```python
from build123d import *

# Parameters (mm, degrees)
SKETCH056_W             = 126
SKETCH056_H             = 25
SKETCH056_R             = 2.2
PAD024_DEPTH            = 3
SKETCH057_W             = 12.4
SKETCH057_H             = 4
PAD025_DEPTH            = 21.5
SKETCH058_R             = 2.2
POCKET031_DEPTH         = 10.609
CHAMFER023_SIZE         = 1
BODY012_ROLL_ANGLE      = 90
BODY012_PLACEMENT_ANGLE = 180


with BuildPart() as part:
    # Sketch056 → Pad024 (new body)
    with BuildSketch(Plane.XY):
        Rectangle(SKETCH056_W, SKETCH056_H)
        with Locations((-53, 0.726)):
            Circle(SKETCH056_R, mode=Mode.SUBTRACT)
        with Locations((53, 0.726)):
            Circle(SKETCH056_R, mode=Mode.SUBTRACT)
    extrude(amount=PAD024_DEPTH)

    # Sketch057 (on Face8 of Pad024) → Pad025 (join)
    with BuildSketch(Plane.XY.offset(3)):
        with Locations((-38.154, -3.892)):
            Rectangle(SKETCH057_W, SKETCH057_H)
        with Locations((38.154, -3.892)):
            Rectangle(SKETCH057_W, SKETCH057_H)
    extrude(amount=PAD025_DEPTH)

    # Sketch058 (on Face12 of Pad025) → Pocket031 (cut, through all)
    with BuildSketch(Plane(origin=(0, -1.892, 0), x_dir=(-1, 0, 0), z_dir=(0, 1, 0))):
        with Locations((-38.154, 18.3)):
            Circle(SKETCH058_R)
        with Locations((38.154, 18.3)):
            Circle(SKETCH058_R)
    extrude(amount=-POCKET031_DEPTH, mode=Mode.SUBTRACT)

    # Chamfer023
    chamfer023_edges = [part.edges().sort_by_distance(p)[0] for p in [
        (0, 12.5, 0),
        (63, 0, 0),
        (0, -12.5, 0),
        (-63, 0, 0),
        (50.8, 0.726, 0),
        (-55.2, 0.726, 0),
    ]]
    chamfer(chamfer023_edges, length=CHAMFER023_SIZE)


with BuildPart() as part_1:
    # Body012 roll: moved
    add(part.part.rotate(Axis((0, 0, 0), (1, 0, 0)), BODY012_ROLL_ANGLE))


with BuildPart() as part_2:
    # Body012 placement: moved
    add(part_1.part.moved(Location((0, -143.1, -77.85))).rotate(Axis((0, -143.1, -77.85), (0, 0, 1)), BODY012_PLACEMENT_ANGLE))


solid = part_2.part
```
Input: part model. Units: mm. Frame: model coordinates. A direction names the side the tool comes from. Round coordinates to 2 decimals unless told otherwise and drop trailing zeros. Order: outer loops, then holes, each group sorted by start corner. A loop starts at its lowest first (then second) coordinate and runs counter-clockwise, first axis right, second up. Notation, with made-up numbers: (58.5, -35.75) - (87.5, -35.75) arc R25 cw to (87.5, -0.75) - close; hole circle Ø7 at (67, 51). An arc over 180 degrees is marked (long way). One line per question, with ' | ' between items. Start each with the question number.
1) Contact query for flat-ended pins moving along their axis: P1, Ø4.5, axis at y = -130.5, z = -81, coming from the -X side; P2, Ø5.5, axis at x = -38.154, y = -124.8, coming from the +Z side; P3, Ø5.5, axis at x = 53, z = -77.124, coming from the +Y side; P4, Ø2, axis at y = -122, z = -86.5, coming from the -X side. Output: stop coordinate, or through.
2) Pull-direction query (Y, two-part tool) for faces 1 (the cylindrical face through (36.41, -126.14, -81.71)), 2 (the cylindrical face through (-40.35, -124.7, -81.71)), 3 (the flat face through (-38, -118.6, -82)), 4 (the cylindrical face through (53.48, -141.11, -79.27)); classes: +Y half, -Y half, draft (parallel to the pull), parting line (faces both ways), or undercut.
3) Cut plane C-C, the plane z = -81.75. Return the cut outline in (x, y), then the cut area to 3 significant figures.
4) Set-up query: faces 5 (the flat face through (38, -130, -83.742)), 6 (the flat face through (38, -130, -79.742)), 7 (the flat face through (-31.954, -130, -82)). Return all of +Z, -Z, +X, -X, +Y, -Y with unobstructed straight access to the full face (end or side cutting, diameter ignored); none if empty.
5) Cut plane D-D, the plane x = 27. Return the cut outline in (y, z).
6) Ray query, probe 1 along Z at (x, y) = (53, -140.9); probe 2 along Y at (x, z) = (36, -79.5); probe 3 along Z at (x, y) = (-42.5, -137.5). Return the intervals inside material, ascending.
7) Cut plane B-B, the plane x = 53. Return the cut outline in (y, z), then the cut area to 3 significant figures.
8) Cut plane A-A, the plane y = -121.5. Return the cut outline in (x, z).
Worked out:
1) P1: stops at x = -44.35 | P2: stops at z = -79.74 | P3: stops at y = -140.1 | P4: passes through
2) face 1: undercut | face 2: undercut | face 3: +Y half | face 4: draft
3) outline: (-63, -142.1) - (-62, -143.1) - (62, -143.1) - (63, -142.1) - (63, -140.1) - (44.35, -140.1) - (44.35, -118.6) - (31.95, -118.6) - (31.95, -140.1) - (-31.95, -140.1) - (-31.95, -118.6) - (-44.35, -118.6) - (-44.35, -140.1) - (-63, -140.1) - close; hole circle Ø4.4 at (-38.15, -124.8); hole circle Ø4.4 at (38.15, -124.8) | area: 880 mm^2
4) face 5: -Z, +X, -X, +Y | face 6: +Z, +X, -X, +Y | face 7: +Z, -Z, +Y
5) outline: (-143.1, -89.35) - (-142.1, -90.35) - (-140.1, -90.35) - (-140.1, -65.35) - (-142.1, -65.35) - (-143.1, -66.35) - close
6) probe 1: z = -90.35 to -79.32, -74.92 to -65.35 | probe 2: y = -143.1 to -140.1 | probe 3: z = -83.74 to -79.74
7) outline: (-143.1, -89.35) - (-142.1, -90.35) - (-140.1, -90.35) - (-140.1, -79.32) - (-142.1, -79.32) - (-143.1, -80.32) - close; (-143.1, -73.92) - (-142.1, -74.92) - (-140.1, -74.92) - (-140.1, -65.35) - (-142.1, -65.35) - (-143.1, -66.35) - close | area: 59.8 mm^2
8) outline: (-44.35, -83.74) - (-31.95, -83.74) - (-31.95, -79.74) - (-44.35, -79.74) - close; (31.95, -83.74) - (44.35, -83.74) - (44.35, -79.74) - (31.95, -79.74) - close
